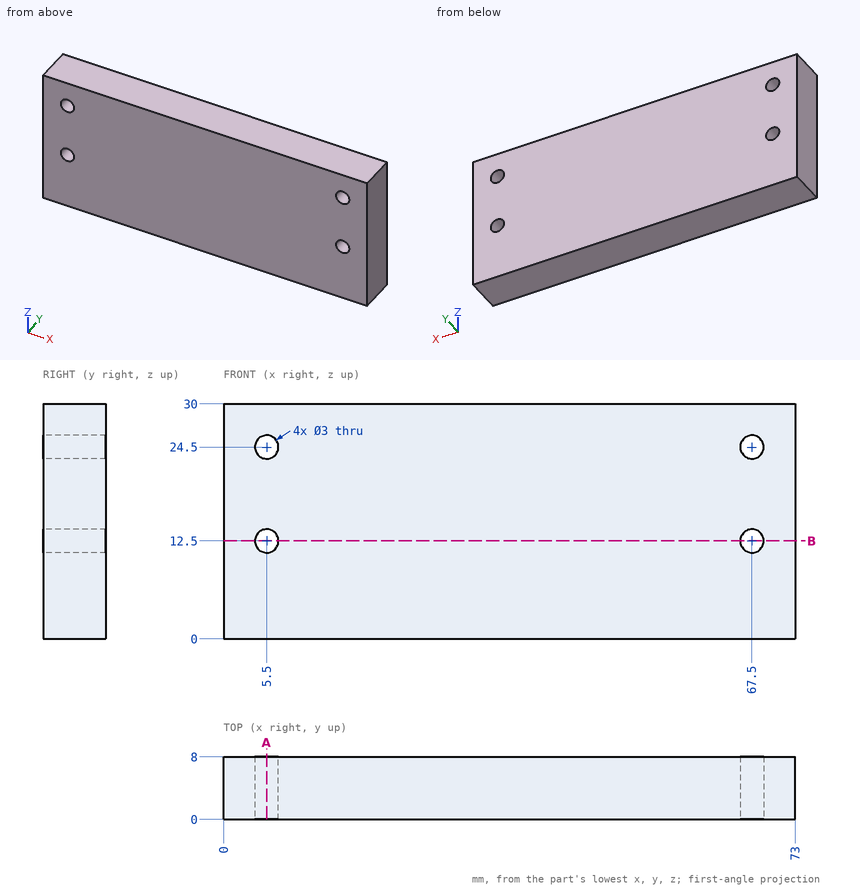
Check sheet for the drawn part. Datum: minimum x, y, z corner. Units: mm. Give positions to 0.01 mm unless a question says otherwise; leave off trailing zeros. Write each loop counter-clockwise with the first axis right and the second up, starting at its lowest first coordinate (ties: lowest second). Pieces come first, ordered by that corner, then holes. Notation, with made-up numbers: (-31, 28.5) - (26, 28.5) arc R28 cw to (26, 49.5) - close; hole circle Ø3 at (72.25, 58). An arc over 180 degrees is marked (long way). Put each result on its own line as item: value.
1. Sectioned sample at B-B, the plane z = 12.5. Enter the section's corners in (x, y), plus the area to 3 significant figures.
Ans:
outline: (0, 0) - (4, 0) - (4, 8) - (0, 8) - close; (7, 0) - (66, 0) - (66, 8) - (7, 8) - close; (69, 0) - (73, 0) - (73, 8) - (69, 8) - close
area: 536 mm²
2. Thickness scan on line 1 (Z direction, x = 67.5, y = 2.75). Record the ranges inside material, lowest first.
Ans:
line 1: z = 0 to 11, 14 to 23, 26 to 30
3. Sectioned sample at A-A, the plane x = 5.5. Enter the section's corners in (y, z).
Ans:
outline: (0, 0) - (8, 0) - (8, 11) - (0, 11) - close; (0, 14) - (8, 14) - (8, 23) - (0, 23) - close; (0, 26) - (8, 26) - (8, 30) - (0, 30) - close
4. Go/stop test with flat-tipped pins: pin 1 (12 mm diameter, centred on x = 51, z = 18, fed in from -Y); pin 2 (1.8 mm diameter, centred on x = 67.5, z = 24.5, fed in from -Y). Record where each tip stops, or that it passes through.
Ans:
pin 1: stops at y = 0
pin 2: passes through
